Build history of the part. All positions in model axes, mm. Face numbers are marked on the shaded views. A direction names the side the tool comes from. Round coordinates to 2 decimals unless told otherwise and drop trailing zeros. Write each loop counter-clockwise with the first axis right and the second up, starting at its lowest first coordinate (ties: lowest second). Pieces come first, ordered by that corner, then holes. Notation, with made-up numbers: (20.5, 43.25) -> (42.5, 43.25) arc R21 cw to (42.5, 70.25) -> close; hole circle Ø5 at (-18.75, 37). An arc over 180 degrees is marked (long way). Answer in a Markdown table with one row per item.
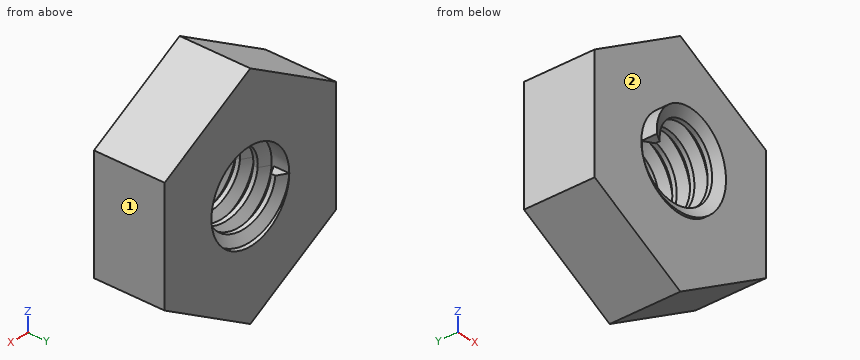
```python
from build123d import *

# Parameters (mm, degrees)
SKETCH1_R           = 1.984375
BOSS_EXTRUDE1_DEPTH = 3.175
THREAD1_PITCH       = 0.79375


with BuildPart() as part:
    # Sketch1 → Boss-Extrude1 (new body)
    with BuildSketch(Plane(origin=(0, 0, 0), x_dir=(1, 0, 0), z_dir=(0, 1, 0))):
        Polygon((0, 5.040989538), (-4.365625, 2.520494769), (-4.365625, -2.520494769), (0, -5.040989538), (4.365625, -2.520494769), (4.365625, 2.520494769), align=None)
        with Locations(Location((0, 0, 0), (0, 0, 270))):
            Circle(SKETCH1_R, mode=Mode.SUBTRACT)
    extrude(amount=BOSS_EXTRUDE1_DEPTH)

    # Thread1: the profile of Thread Profile1 profile screwed along a right-hand helix of 4 turns, 8 arcs to a turn; built about Z, then put on its axis
    thread1_z = Axis((0, 0, 0), (0, 0, 1))
    thread1_corners = [(1.984675, 0, -0.000173205), (1.984675, 0, 0.694704453), (1.554745212, 0, 0.446484374), (1.554745212, 0, 0.248046874)]
    with BuildLine(mode=Mode.PRIVATE) as thread1_profile:
        Line(thread1_corners[0], thread1_corners[1])
        Line(thread1_corners[1], thread1_corners[2])
        Line(thread1_corners[2], thread1_corners[3])
        Line(thread1_corners[3], thread1_corners[0])
    thread1_cap = Face(thread1_profile.wire())
    thread1_turn_angles = [0, 22.5, 45, 67.5, 90, 112.5, 135, 157.5, 180, 202.5, 225, 247.5, 270, 292.5, 315, 337.5, 360]
    thread1_turn_weights = [1, 0.9238795325112867, 1, 0.9238795325112867, 1, 0.9238795325112867, 1, 0.9238795325112867, 1, 0.9238795325112867, 1, 0.9238795325112867, 1, 0.9238795325112867, 1, 0.9238795325112867, 1]
    thread1_turn_rails = [Edge.make_bspline([Vector(p[0], p[1], 0).rotate(thread1_z, thread1_turn_angles[k]) / thread1_turn_weights[k] + Vector(0, 0, p[2] + THREAD1_PITCH * thread1_turn_angles[k] / 360) for k in range(17)], [0, 0, 0, 1, 1, 2, 2, 3, 3, 4, 4, 5, 5, 6, 6, 7, 7, 8, 8, 8], 2, thread1_turn_weights) for p in thread1_corners]
    thread1_turn_sides = [Face.make_surface_from_curves(thread1_turn_rails[p[0]], thread1_turn_rails[p[1]]) for p in [(0, 1), (1, 2), (2, 3), (3, 0)]]
    thread1 = Plane(origin=(0, 3.175, 0), x_dir=(-1, 0, 0), z_dir=(0, -1, 0)) * Solid(Shell([*[p.moved(Location((0, 0, THREAD1_PITCH * i))) for i in range(4) for p in thread1_turn_sides], thread1_cap, thread1_cap.rotate(thread1_z, 1440).moved(Location((0, 0, THREAD1_PITCH * 1440 / 360)))]))
    add(thread1)


solid = part.part
```
Q1. Wall check: line 1 (Y direction, x = -2.5, z = 3.25) (3 decimals); line 2 (Y direction, x = -1.25, z = 1); line 3 (X direction, y = 0.9, z = -0.25). Give the ranges that are in metal, low to high. Write a range as [from, to].
A:
| item | result |
|---|---|
| line 1 | [0, 3.175] |
| line 2 | [-0.39, -0.14], [0.41, 0.66], [1.2, 1.45], [1.99, 2.25] |
| line 3 | [-4.37, -1.93], [1.53, 4.37] |
Q2. Saw through at B-B on x = -4. Write the cut outline in (y, z) (3 decimals).
A:
| item | result |
|---|---|
| outline | (0, -2.732) -> (3.175, -2.732) -> (3.175, 2.732) -> (0, 2.732) -> close |
Q3. Saw through at A-A on z = -2.25. Write the cut outline in (x, y) (3 decimals).
A:
| item | result |
|---|---|
| outline | (-4.366, 0) -> (4.366, 0) -> (4.366, 3.175) -> (-4.366, 3.175) -> close |
Q4. Which spindle directions (+Z, -Z, +X, -X, +Y, -Y) get a long thin tool onto all of the face, cutting with end or side? Do the marked faces 1 and 2. Say none if no direction does.
A:
| item | result |
|---|---|
| face 1 | +Z, -Z, +X, +Y, -Y |
| face 2 | -Y |
Q5. Drop flat-ended pins along their axis: P1, Ø1.5, axis at x = -0.5, y = 0.5, coming from the +Z side; P2, Ø2, axis at x = 0.5, z = 0.5, coming from the +Y side. Give the stop position or say it passes through.
A:
| item | result |
|---|---|
| P1 | z = 5.04 |
| P2 | y = 2.53 |
